Input: part model. Units: mm. Frame: model coordinates. Face numbers are marked on the shaded views. A direction names the side the tool comes from. Round coordinates to 2 decimals unless told otherwise and drop trailing zeros. Order: outer loops, then holes, each group sorted by start corner. A loop starts at its lowest first (then second) coordinate and runs counter-clockwise, first axis right, second up. Notation, with made-up numbers: (75, 47) -> (105, 47) arc R7 ccw to (105, 55) -> close; hole circle Ø4 at (17, 35). An arc over 180 degrees is marked (long way). Use a Markdown table: item, result.
Autodesk Inventor part; units mm, degrees
ref_plane "YZ Plane" through (0, 0, 0) normal (1, 0, 0) x (0, 1, 0)
ref_plane "XZ Plane" through (0, 0, 0) normal (0, 1, 0) x (-1, 0, 0)
ref_plane "XY Plane" through (0, 0, 0) normal (0, 0, 1) x (1, 0, 0)
sketch "Эскиз1" plane through (0, 0, 0) normal (0, 0, 1) x (1, 0, 0)
  line L0 (-9, 13.4) -> (9, 13.4)
  line L1 (21, -19.4) -> (-21, -19.4)
  line L2 (-21, -19.4) -> (-21, -13.4)
  line L3 (-9, 13.4) -> (-9, -13.4)
  line L4 (9, 13.4) -> (9, -13.4)
  line L5 (21, -19.4) -> (21, -13.4)
  line L6 (-21, -13.4) -> (-9, -13.4)
  line L7 (9, -13.4) -> (21, -13.4)
  point P0 (0, 0)
  point P1 (-9, 0)
  point P2 (0, -19.4)
  dimension "d0" = 42
  dimension "d2" = 18
  dimension "d3" = 9
  dimension "d6" = 6
  dimension "d7" = 32.8
extrude "Выдавливание1" add sketch "Эскиз1" along normal mid plane 14
sketch "Эскиз3" plane through (0, 0, 7) normal (0, 0, 1) x (1, 0, 0)
  line L0 (-21, -19.4) -> (21, -19.4)
  point P0 (0, 0)
  point P1 (0, 0.6)
  dimension "d12" = 20
hole "Отверстие1" at (0, 0.6, 7) direction (0, 0, -1) diameter 8.2 end through all
sketch "Эскиз4" plane through (0, 0, 7) normal (0, 0, 1) x (1, 0, 0)
  line L0 (-9, 13.4) -> (9, 13.4)
  line L1 (-0.75, 13.4) -> (-0.75, 4.6308)
  circle A0 centre (0, 0.6) radius 4.1
  line L2 (0.75, 13.4) -> (0.75, 4.6308)
  point P0 (0, 0)
  dimension "d20" = 1.5
  dimension "d21" = 0.75
extrude "Выдавливание2" cut sketch "Эскиз4" against normal blind 14 contours L0 L2 A0 L1
sketch "Эскиз6" plane through (9, -13.4, 7) normal (0, 1, 0) x (1, 0, 0)
  line L0 (12, 14) -> (12, 0)
  line L1 (0, 14) -> (12, 14)
  point P0 (-9, 7)
  point P1 (6, 7)
  point P2 (12, 7)
  point P3 (6, 14)
hole "Отверстие3" at (15, -13.4, 0) direction (0, -1, 0) diameter 5.5 end through all
sketch "Эскиз7" plane through (-21, -13.4, 7) normal (0, 1, 0) x (1, 0, 0)
  line L0 (0, 14) -> (12, 14)
  line L1 (0, 0) -> (0, 14)
  point P0 (21, 7)
  point P1 (6, 7)
  point P2 (6, 14)
  point P3 (0, 7)
hole "Отверстие4" at (-15, -13.4, 0) direction (0, -1, 0) diameter 5.5 end through all
sketch "Эскиз8" plane through (9, -13.4, 7) normal (1, 0, 0) x (0, 0, -1)
  line L0 (14, 26.8) -> (0, 26.8)
  point P0 (7, 13.4)
  point P1 (7, 22.95)
  point P2 (7, 26.8)
  dimension "d50" = 3.85
sketch "Эскиз9" plane through (9, -13.4, 7) normal (1, 0, 0) x (0, 0, -1)
  point P0 (7, 13.4)
hole "Отверстие5" at (9, 9.55, 0) direction (-1, 0, 0) diameter 4.1 end through all
thread "Резьба2"
sketch "Эскиз10" plane through (9, -13.4, 7) normal (1, 0, 0) x (0, 0, -1)
  circle A0 centre (7, 22.95) radius 2.5
  line L0 (14, 26.8) -> (0, 26.8)
  point P0 (7, 13.4)
  point P1 (7, 26.8)
  dimension "d60" = 5
  dimension "d61" = 3.85
extrude "Выдавливание3" cut sketch "Эскиз10" against normal blind 5
chamfer "Фаска1" distance 1 angle 45 8 edges at (0, -3.5, 7) (-9, 9.55, 2.05) (-15, -19.4, -2.75) (15, -19.4, -2.75) (0, -3.5, -7) (15, -13.4, -2.75) (-15, -13.4, -2.75) (9, 9.55, 2.5)
properties part number "SK10"
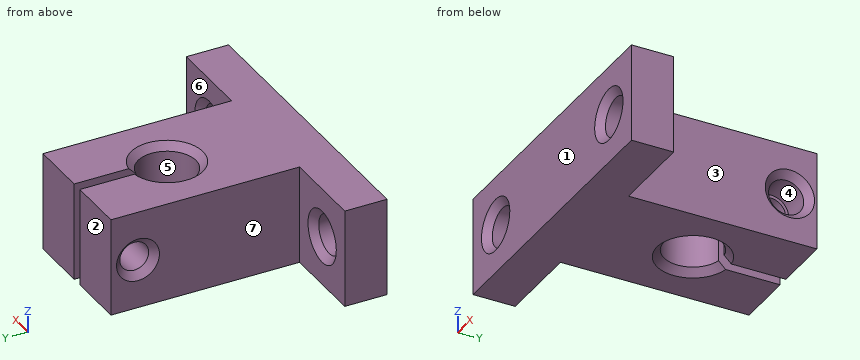
1) Contact query for flat-ended pins moving along their axis: P1, Ø4.5, axis at x = -15, z = 0, coming from the -Y side; P2, Ø10, axis at x = 11, y = -1, coming from the -Z side; P3, Ø2.5, axis at y = 7, z = -2, coming from the -X side; P4, Ø5.5, axis at y = 9.55, z = 0, coming from the +X side. Output: stop coordinate, or through.
Answer key:
| item | result |
|---|---|
| P1 | passes through |
| P2 | stops at z = -7 |
| P3 | stops at x = -9 |
| P4 | stops at x = 8.25 |
2) Cut plane C-C on y = 9.55. Return loops of the section in (x, z).
Answer key:
| item | result |
|---|---|
| outline | (-9, -7) -> (-0.75, -7) -> (-0.75, -2.05) -> (-8, -2.05) -> (-9, -3.05) -> close; (-9, 3.05) -> (-8, 2.05) -> (-0.75, 2.05) -> (-0.75, 7) -> (-9, 7) -> close; (0.75, -7) -> (9, -7) -> (9, -3.5) -> (8, -2.5) -> (4, -2.5) -> (4, -2.05) -> (0.75, -2.05) -> close; (0.75, 2.05) -> (4, 2.05) -> (4, 2.5) -> (8, 2.5) -> (9, 3.5) -> (9, 7) -> (0.75, 7) -> close |
3) Cut plane D-D on z = 0. State how many separate pieces and enclosed holes the cut face has, and give its area (3 significant figures).
Answer key:
| item | result |
|---|---|
| separate pieces | 5 |
| enclosed holes | 0 |
| area | 524 mm^2 |
4) Cut plane A-A on y = 0.6. Return loops of the section in (x, z), and give its area (3 significant figures).
Answer key:
| item | result |
|---|---|
| outline | (-9, -7) -> (-5.1, -7) -> (-4.1, -6) -> (-4.1, 6) -> (-5.1, 7) -> (-9, 7) -> close; (4.1, -6) -> (5.1, -7) -> (9, -7) -> (9, 7) -> (5.1, 7) -> (4.1, 6) -> close |
| area | 135 mm^2 |
5) Set-up query: the marked faces 5, 6 and 7. Return all of +Z, -Z, +X, -X, +Y, -Y with unobstructed straight access to the full face (end or side cutting, diameter ignored); none if empty.
Answer key:
| item | result |
|---|---|
| face 5 | +Z, -Z |
| face 6 | +Z, -Z, +X, +Y |
| face 7 | +Z, -Z, -X, +Y |
6) Draft query along Y for the marked faces 1, 2, 3 and 4. Return one class per face: released by +Y, released by -Y, zero draft, split by the parting line, or undercut.
Answer key:
| item | result |
|---|---|
| face 1 | released by -Y |
| face 2 | released by +Y |
| face 3 | zero draft |
| face 4 | undercut |
7) Ray query, probe 1 along X at (y, z) = (-15.75, 0); probe 2 along Z at (x, y) = (-15, -17); probe 3 along X at (y, z) = (5.5, 4.25). Return the intervals inside material, ascending.
Answer key:
| item | result |
|---|---|
| probe 1 | x = -21 to -17.75, -12.25 to 12.25, 17.75 to 21 |
| probe 2 | z = -7 to -2.75, 2.75 to 7 |
| probe 3 | x = -9 to -0.75, 0.75 to 9 |
8) Cut plane B-B on x = 15. Return loops of the section in (y, z), and give its area (3 significant figures).
Answer key:
| item | result |
|---|---|
| outline | (-19.4, -7) -> (-13.4, -7) -> (-13.4, -3.75) -> (-14.4, -2.75) -> (-18.4, -2.75) -> (-19.4, -3.75) -> close; (-19.4, 3.75) -> (-18.4, 2.75) -> (-14.4, 2.75) -> (-13.4, 3.75) -> (-13.4, 7) -> (-19.4, 7) -> close |
| area | 49.0 mm^2 |
